The figure shows three views and two pictorial views of one solid part (mm, origin at its lowest corner). Answer the questions. Coordinates: 2 decimals unless noted, no trailing zeros. Write each loop counter-clockwise with the first axis right and the second up, starting at its lowest first coordinate (ties: lowest second). Pieces come first, ordered by that corner, then holes.
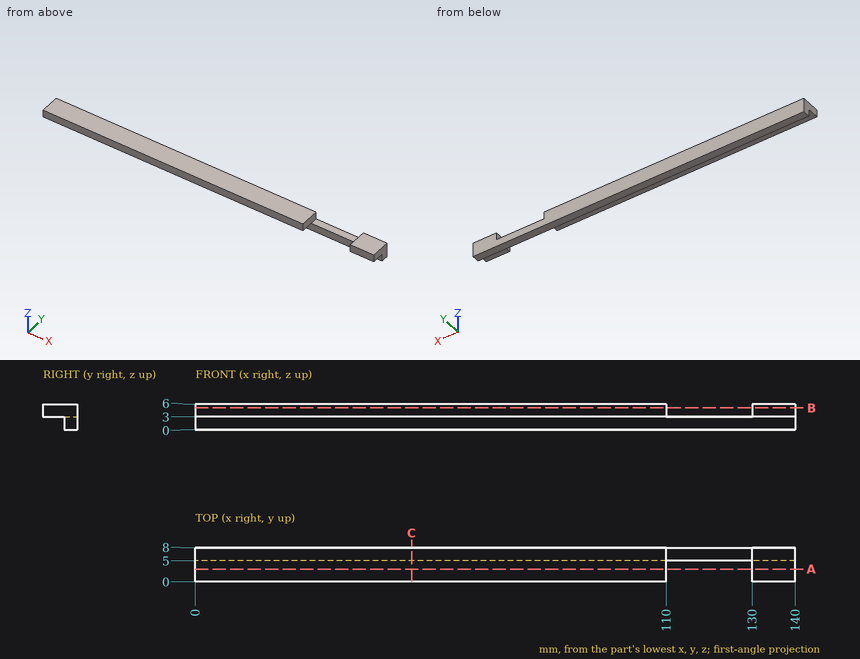
Q1. Given pin 1 (1.5 mm diameter, centred on x = 85, z = 1.5, fed in from -Y); pin 2 (2.5 mm diameter, centred on y = 6, z = 5, fed in from -X); pin 3 (2.5 mm diameter, centred on x = 120.5, y = 6, fed in from +Z), each flat-ended and moving along its own axis, determine where each tip first touches the part or whether it passes through.
Answers below:
pin 1: stops at y = 5
pin 2: stops at x = 0
pin 3: stops at z = 3
Q2. The part is cut by section B-B, the plane z = 5.1. Write down the section's boundary in (x, y).
Answers below:
outline: (0, 0) - (110, 0) - (110, 8) - (0, 8) - close; (130, 0) - (140, 0) - (140, 8) - (130, 8) - close
Q3. The part is cut by section C-C, the plane x = 50.5. Write down the section's boundary in (y, z), then the cut area to 3 significant figures.
Answers below:
outline: (0, 3) - (5, 3) - (5, 0) - (8, 0) - (8, 6) - (0, 6) - close
area: 33.0 mm2
Q4. Find the intervals of material crossed by probe 1 along X at (y, z) = (3, 3.7); probe 2 along Y at (x, z) = (18, 0.45); probe 3 along Z at (x, y) = (95.5, 3), in increasing order.
Answers below:
probe 1: x = 0 to 110, 130 to 140
probe 2: y = 5 to 8
probe 3: z = 3 to 6
Q5. The part is cut by section A-A, the plane y = 3. Write down the section's boundary in (x, z), then the cut area to 3 significant figures.
Answers below:
outline: (0, 3) - (110, 3) - (110, 6) - (0, 6) - close; (130, 3) - (140, 3) - (140, 6) - (130, 6) - close
area: 360 mm2
